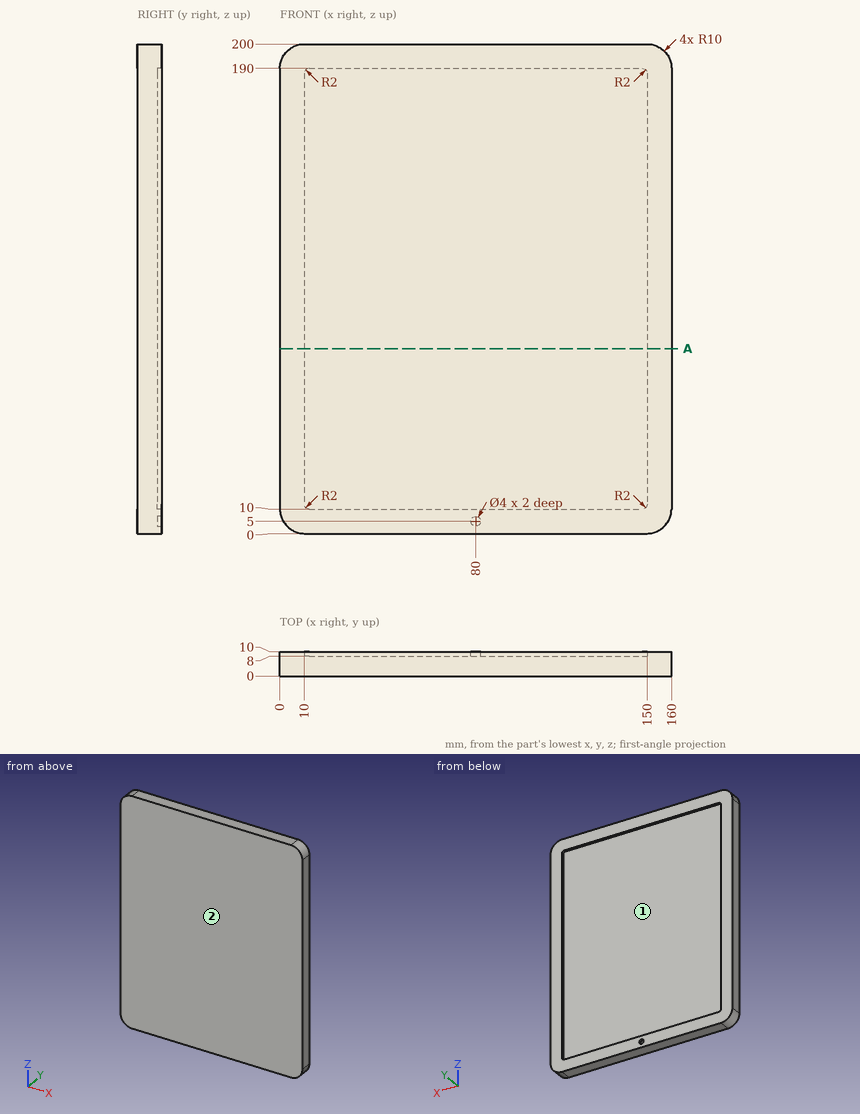
Verification items for this drawing (mm, ordinates from the low corner). Round coordinates to 2 decimals unless told otherwise and drop trailing zeros. Loops run counter-clockwise (first coordinate to the right, second up) from the corner with the lowest first, then second, coordinate; pieces in that order, holes last. Notation, with made-up numbers: M 78.5,-5 L 124.5,-5 A6 ccw 124.5,2 Z; hole C -31,-34.5 d9. An arc over 180 degrees is marked long. Answer as a JSON object with one key per item and string values.
1. Scan lines: line 1 (Z direction, x = 32.5, y = 9); line 2 (X direction, y = 9.25, z = 145.5); line 3 (Y direction, x = 59.5, z = 178). Record each from-to range of solid material in increasing order.
Reply:
{"line 1": "z = 0 to 10, 190 to 200", "line 2": "x = 0 to 10, 150 to 160", "line 3": "y = 0 to 8"}
2. Section check A-A (z = 75.5). Record the boundary of the cut face in (x, y).
Reply:
{"outline": "M 0,0 L 160,0 L 160,10 L 150,10 L 150,8 L 10,8 L 10,10 L 0,10 Z"}
3. Gauge pin test, flat ends, axial feed: P1, Ø5, axis at x = 80, z = 5, coming from the +Y side; P2, Ø5, axis at x = 126, z = 149, coming from the +Y side. Record the tip position at first contact, or that the pin passes through.
Reply:
{"P1": "stops at y = 10", "P2": "stops at y = 8"}
4. Mould release check, pull along Z, two halves, no side actions. Record for the marked faces 1 and 2: pulls with the +Z half, pulls with the -Z half, needs draft (parallel to the pull), parting line crosses it, or undercut.
Reply:
{"face 1": "undercut", "face 2": "needs draft"}
